```python
from build123d import *

# Parameters (mm, degrees)
ROBOTCHASSIS1_START = 54.665073828
ROBOTCHASSIS1_DEPTH = 3.000000026
SKETCH1_R           = 1.763889566
BOSS_EXTRUDE2_DEPTH = 3.000000026


# Read off the part's stored shape, not the designer's step: RobotChassis1
with BuildPart() as part:
    # RobotChassis1 outline → RobotChassis1 (new body)
    with BuildSketch(Plane.XY.offset(ROBOTCHASSIS1_START)):
        Polygon((78.391484289, 73.860644449), (78.215099244, 74.037033219), (78.038699298, 74.142797936), (77.826834588, 74.248562653), (77.615297704, 74.354670097), (77.403775721, 74.424951424), (77.191881209, 74.460434814), (51.474607854, 74.460434814), (51.474607854, 76.471339066), (46.958781152, 76.471339066), (46.782381206, 76.435855676), (46.605996161, 76.400715013), (46.46509078, 76.330094684), (46.323842673, 76.224326242), (46.182937293, 76.118561525), (46.11232069, 75.977313419), (46.006552248, 75.800920923), (45.971072583, 75.624535878), (45.971072583, 61.301893641), (46.006552248, 61.125501145), (46.11232069, 60.9491161), (46.182937293, 60.807867993), (46.323842673, 60.702103276), (46.46509078, 60.59633856), (46.605996161, 60.525714506), (46.782381206, 60.490231116), (46.958781152, 60.455090453), (51.474607854, 60.455090453), (51.474607854, 62.46599098), (77.191881209, 62.46599098), (77.403775721, 62.501131643), (77.826834588, 62.64237975), (78.038699298, 62.78328513), (78.215099244, 62.889392574), (78.391484289, 63.030297954), (78.53238967, 63.206686725), (78.673637776, 63.383075495), (78.779391317, 63.594947655), (78.920654326, 64.018006523), (78.955791264, 64.229882408), (78.955791264, 72.69654711), (78.920654326, 72.908076544), (78.850022822, 73.119948704), (78.779391317, 73.331478138), (78.673637776, 73.507866908), (78.53238967, 73.719396342), align=None)
        Polygon((58.177388578, 70.19161721), (58.388910561, 70.156476547), (58.600447445, 70.085852493), (58.77683249, 70.01522844), (58.953217535, 69.909463723), (59.12960258, 69.768562068), (59.270850687, 69.627310236), (59.412098794, 69.45091774), (59.517867236, 69.274532695), (59.58849874, 69.063003261), (59.658772616, 68.886614491), (59.694252281, 68.67474233), (59.729404121, 68.463212897), (59.694252281, 68.251340736), (59.658772616, 68.039811303), (59.58849874, 67.828281869), (59.517867236, 67.651893098), (59.412098794, 67.475504328), (59.270850687, 67.299111832), (59.12960258, 67.157867451), (58.953217535, 67.016619344), (58.77683249, 66.910854627), (58.600447445, 66.840230574), (58.388910561, 66.769949247), (58.177388578, 66.734465857), (57.965508967, 66.699325193), (54.966903596, 66.699325193), (54.755366712, 66.734465857), (54.543502002, 66.769949247), (54.331965118, 66.840230574), (54.155580072, 66.910854627), (53.979195027, 67.016619344), (53.802795081, 67.157867451), (53.661546974, 67.299111832), (53.520641594, 67.475504328), (53.414873152, 67.651893098), (53.344256549, 67.828281869), (53.273639946, 68.039811303), (53.238488107, 68.251340736), (53.203008442, 68.463212897), (53.238488107, 68.67474233), (53.273639946, 68.886614491), (53.344256549, 69.063003261), (53.414873152, 69.274532695), (53.520641594, 69.45091774), (53.661546974, 69.627310236), (53.802795081, 69.768562068), (53.979195027, 69.909463723), (54.155580072, 70.01522844), (54.331965118, 70.085852493), (54.543502002, 70.156476547), (54.755366712, 70.19161721), (54.966903596, 70.227104325), (57.965508967, 70.227104325), align=None, mode=Mode.SUBTRACT)
        Polygon((74.581555395, 70.085852493), (74.79309228, 70.01522844), (74.969462423, 69.909463723), (75.11071053, 69.768562068), (75.287110477, 69.627310236), (75.49863246, 69.274532695), (75.604400902, 69.063003261), (75.675017505, 68.886614491), (75.710169344, 68.67474233), (75.710169344, 68.251340736), (75.675017505, 68.039811303), (75.604400902, 67.828281869), (75.287110477, 67.299111832), (75.11071053, 67.157867451), (74.969462423, 67.016619344), (74.79309228, 66.910854627), (74.581555395, 66.840230574), (74.369675784, 66.769949247), (74.158153801, 66.734465857), (73.94627419, 66.699325193), (73.769889145, 66.734465857), (73.558352261, 66.769949247), (73.346830278, 66.840230574), (73.134950667, 66.910854627), (72.958565621, 67.016619344), (72.817660241, 67.157867451), (72.641275196, 67.299111832), (72.535164027, 67.475504328), (72.323627143, 67.828281869), (72.25301054, 68.039811303), (72.217873602, 68.251340736), (72.217873602, 68.67474233), (72.25301054, 68.886614491), (72.323627143, 69.063003261), (72.429395585, 69.274532695), (72.535164027, 69.45091774), (72.641275196, 69.627310236), (72.817660241, 69.768562068), (72.958565621, 69.909463723), (73.134950667, 70.01522844), (73.346830278, 70.085852493), (73.558352261, 70.156476547), (73.769889145, 70.19161721), (73.94627419, 70.227104325), (74.158153801, 70.19161721), (74.369675784, 70.156476547), align=None, mode=Mode.SUBTRACT)
    extrude(amount=ROBOTCHASSIS1_DEPTH)


with BuildPart() as body_2:
    # Sketch1 → Boss-Extrude2 (new body)
    with BuildSketch(Plane.XY.offset(57.665073854)):
        with BuildLine():
            Line((51.474607854, 74.460434814), (77.191881209, 74.460434814))
            ThreePointArc((77.191881209, 74.460434814), (78.378212032, 73.882870615), (78.955791264, 72.69654711))
            Line((78.955791264, 72.69654711), (78.955791264, 64.229882408))
            ThreePointArc((78.955791264, 64.229882408), (78.386068245, 63.035701388), (77.191881209, 62.46599098))
            Line((77.191881209, 62.46599098), (51.474607854, 62.46599098))
            Line((51.474607854, 62.46599098), (51.474607854, 60.455090453))
            Line((51.474607854, 60.455090453), (46.958781152, 60.455090453))
            ThreePointArc((46.958781152, 60.455090453), (46.319168008, 60.708479372), (45.971072583, 61.301893641))
            Line((45.971072583, 61.301893641), (45.971072583, 75.624535878))
            ThreePointArc((45.971072583, 75.624535878), (46.319165637, 76.217952912), (46.958781152, 76.471339066))
            Line((46.958781152, 76.471339066), (51.474607854, 76.471339066))
            Line((51.474607854, 76.471339066), (51.474607854, 74.460434814))
        make_face()
        with Locations((73.94627419, 68.463214759)):
            Circle(SKETCH1_R, mode=Mode.SUBTRACT)
        with BuildLine():
            Line((57.965508967, 66.699325193), (54.966903596, 66.699325193))
            ThreePointArc((54.966903596, 66.699325193), (53.20301403, 68.463214759), (54.966903596, 70.227104325))
            Line((54.966903596, 70.227104325), (57.965508967, 70.227104325))
            ThreePointArc((57.965508967, 70.227104325), (59.729398533, 68.463214759), (57.965508967, 66.699325193))
        make_face(mode=Mode.SUBTRACT)
    extrude(amount=-BOSS_EXTRUDE2_DEPTH)


solid = body_2.part
```
Can you work these out from the model? Positions are in its coordinate system, mm. A direction names the side the tool comes from. Coordinates: 2 decimals unless noted, no trailing zeros. Order: outer loops, then holes, each group sorted by start corner. A loop starts at its lowest first (then second) coordinate and runs counter-clockwise, first axis right, second up. Notation, with made-up numbers: (-6.5, 55) -> (37.5, 55) arc R28 cw to (37.5, 80) -> close; hole circle Ø6 at (9.25, -11.75). An arc over 180 degrees is marked (long way). Write each question's results on one line, items separated by ' | '.
Item 1: I'm going to push flat-ended pins straight in: pin 1 Ø1.5 at (x, z) = (64.5, 56.5) entering from +Y; pin 2 Ø0.9 at (x, z) = (55.5, 56) entering from -Y; pin 3 Ø0.6 at (y, z) = (61.5, 56.5) entering from +X; pin 4 Ø4 at (x, y) = (73.95, 68.46) entering from +Z. Where does each tip first touch, or does it pass through?
Results are:
pin 1: y = 74.46 | pin 2: y = 62.47 | pin 3: x = 51.47 | pin 4: z = 57.67
Item 2: I want a section at B-B, the plane y = 67.5. Write out the boundary of the cut face in (x, z).
Results are:
outline: (45.97, 54.67) -> (53.49, 54.67) -> (53.49, 57.67) -> (45.97, 57.67) -> close; (59.44, 54.67) -> (72.47, 54.67) -> (72.47, 57.67) -> (59.44, 57.67) -> close; (75.42, 54.67) -> (78.96, 54.67) -> (78.96, 57.67) -> (75.42, 57.67) -> close
Item 3: I want a section at D-D, the plane x = 68.5. Write out the boundary of the cut face in (y, z), then the cut area to 3 significant figures.
Results are:
outline: (62.47, 54.67) -> (74.46, 54.67) -> (74.46, 57.67) -> (62.47, 57.67) -> close | area: 36.0 mm²
Item 4: I want a section at A-A, the plane x = 56. Write out the boundary of the cut face in (y, z), then the cut area to 3 significant figures.
Results are:
outline: (62.47, 54.67) -> (66.7, 54.67) -> (66.7, 57.67) -> (62.47, 57.67) -> close; (70.23, 54.67) -> (74.46, 54.67) -> (74.46, 57.67) -> (70.23, 57.67) -> close | area: 25.4 mm²
Item 5: If I drill on line 1 along X through (y, z) = (68.5, 55.75); line 2 along X through (y, z) = (67.25, 57.05); line 3 along Y through (x, z) = (58, 55.7), over which ranges is the centre line in solid material (lowest first)?
Results are:
line 1: 45.97 to 53.2, 59.73 to 72.18, 75.71 to 78.96 | line 2: 45.97 to 53.69, 59.25 to 72.67, 75.23 to 78.96 | line 3: 62.47 to 66.7, 70.23 to 74.46
Item 6: If we mould it in two halves opening along X, with no side actions, what happens to faces 1 (the face through (51.475, 75, 56)), 2 (the face through (56, 66.699, 56)), 3 (the face through (64, 74.46, 56))? For each: +X half, -X half, draft (parallel to the pull), parting line (faces both ways), or undercut.
Results are:
face 1: +X half | face 2: undercut | face 3: draft
Item 7: I want a section at C-C, the plane z = 55.8. Write out the boundary of the cut face in (x, y), then the cut area to 3 significant figures.
Results are:
outline: (45.97, 61.3) arc R1.06 ccw to (46.96, 60.46) -> (51.47, 60.46) -> (51.47, 62.47) -> (77.19, 62.47) arc R1.98 ccw to (78.96, 64.23) -> (78.96, 72.7) arc R2.02 ccw to (77.19, 74.46) -> (51.47, 74.46) -> (51.47, 76.47) -> (46.96, 76.47) arc R1.06 ccw to (45.97, 75.62) -> close; hole (54.97, 66.7) -> (57.97, 66.7) arc R1.76 ccw to (57.97, 70.23) -> (54.97, 70.23) arc R1.76 ccw to start; hole circle Ø3.53 at (73.95, 68.46) | area: 386 mm²
Item 8: Which directions (+Z, -Z, +X, -X, +Y, -Y) give clear straight access to the entire face, cutting with the end or side of a thin tool? Please do faces 4 (the face through (78.956, 69, 56)), 5 (the face through (51.475, 61, 56)), 6 (the face through (53.203, 68.424, 56.186)).
Results are:
face 4: +Z, -Z, +X, +Y, -Y | face 5: +Z, -Z, +X, -Y | face 6: +Z, -Z
